Verification items for this drawing (mm, ordinates from the low corner). A direction names the side the tool comes from. Coordinates: 2 decimals unless noted, no trailing zeros. Write each loop counter-clockwise with the first axis right and the second up, starting at its lowest first coordinate (ties: lowest second). Pieces come first, ordered by that corner, then holes. Notation, with made-up numbers: M -7,23 L 46,23 A30 ccw 46,53 Z; hole C 24,53 d8. An arc over 180 degrees is marked long. Write each question's results on one line, items separated by ' | '.
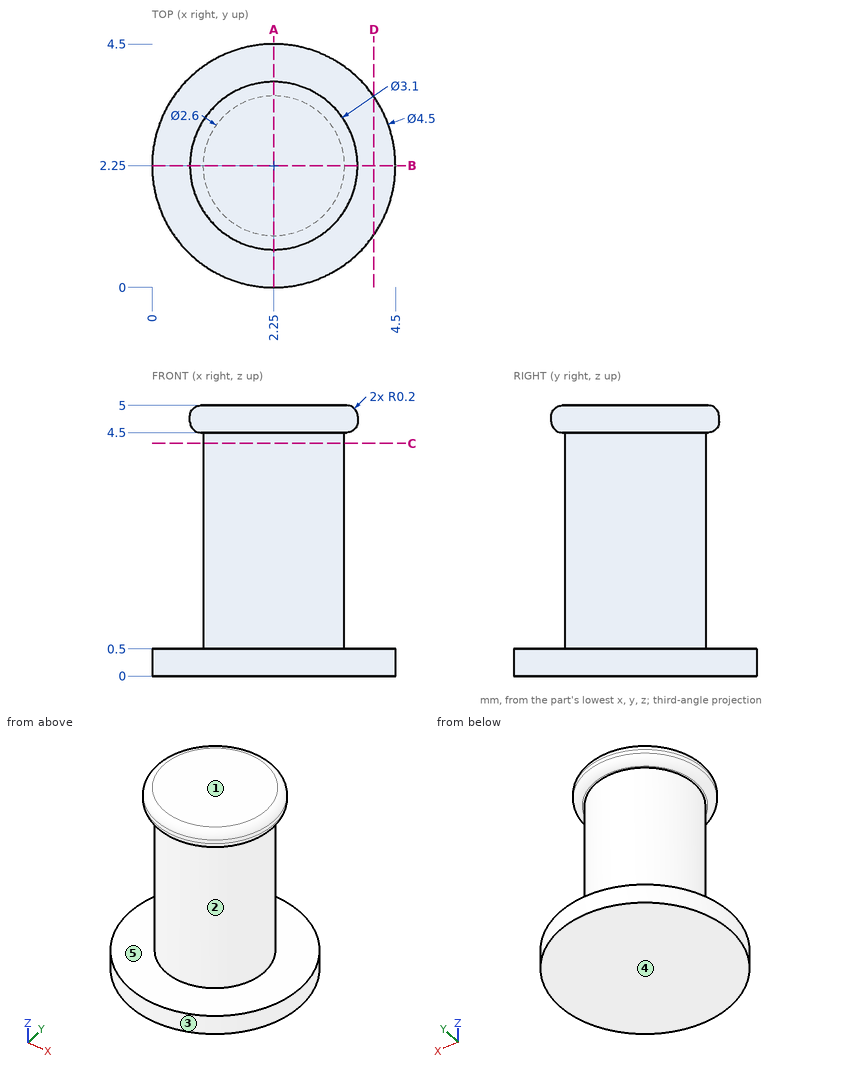
Q1. Sectioned sample at A-A on x = 2.25. Record the cut outline in (y, z).
Geometry check:
outline: M 0,0 L 4.5,0 L 4.5,0.5 L 3.55,0.5 L 3.55,4.5 L 3.6,4.5 A0.2 ccw 3.8,4.7 L 3.8,4.8 A0.2 ccw 3.6,5 L 0.9,5 A0.2 ccw 0.7,4.8 L 0.7,4.7 A0.2 ccw 0.9,4.5 L 0.95,4.5 L 0.95,0.5 L 0,0.5 Z
Q2. Access from +Z, -Z, +X, -X, +Y, -Y to the whole of each face (thin tool, end or side, straight path). Record for the marked faces 4 and 5.
Geometry check:
face 4: -Z, +X, -X, +Y, -Y | face 5: none
Q3. Sectioned sample at D-D on x = 4.1. Record the cut outline in (y, z), and give its area (3 significant figures).
Geometry check:
outline: M 0.97,0 L 3.53,0 L 3.53,0.5 L 0.97,0.5 Z | area: 1.28 mm2
Q4. Sectioned sample at C-C on z = 4.3. Record the cut outline in (x, y).
Geometry check:
outline: C 2.25,2.25 d2.6
Q5. Depth check by flat-ended pin: P1, Ø0.8, axis at x = 2.5, y = 3, coming from the -Z side. Enter the tip coordinate at first touch or a pass-through.
Geometry check:
P1: stops at z = 0
Q6. Mould release check, pull along Z, two halves, no side actions. Record for the marked faces 1, 2 and 3: pulls with the +Z half, pulls with the -Z half, needs draft (parallel to the pull), parting line crosses it, or undercut.
Geometry check:
face 1: pulls with the +Z half | face 2: undercut | face 3: needs draft
Q7. Scan lines: probe 1 along Z at (x, y) = (3.4, 1); probe 2 along X at (y, z) = (0.45, 0.3); probe 3 along X at (y, z) = (2.55, 2.7). Record each from-to range of solid material in increasing order.
Geometry check:
probe 1: z = 0 to 0.5 | probe 2: x = 0.9 to 3.6 | probe 3: x = 0.99 to 3.51
